Input: part model. Units: mm. Frame: model coordinates. Face numbers are marked on the shaded views. Give positions to 0.01 mm unless a question says otherwise; leave off trailing zeros. Loops run counter-clockwise (first coordinate to the right, second up) from the corner with the lowest first, then second, coordinate; pieces in that order, holes last. Notation, with made-up numbers: (54, 80.5) - (75, 80.5) arc R35 ccw to (75, 115.5) - close; hole circle Ø6 at (68.5, -36). An arc over 180 degrees is marked (long way). Answer as a JSON object with one key per item and string values. Group by question number.
(1) Section query C-C (z = -7). Return loops of the section in (x, y) (3 decimals), plus the area to 3 significant figures.
(2) Section query D-D (z = -17.5). Return loops of the section in (x, y), plus the area to 3 significant figures.
(3) Pin query (flat end, axial travel): P1, Ø3, axis at x = 0, z = 0, coming from the -Y side; P2, Ø1, axis at x = 3.5, y = 6.5, coming from the +Z side; P3, Ø3, axis at x = -15.5, z = 3.5, coming from the -Y side; P4, Ø4, axis at y = 4, z = 4, coming from the +X side. Return the tip coordinate at first contact, or that it passes through.
(4) Section query A-A (y = 3.5). Return loops of the section in (x, z).
(5) Material intervals for L1, parallel to X at y = 5.75, z = 0; L2, parallel to X at y = 2.75, z = 0; L3, parallel to Y at x = -14.5, z = -1, sorted ascending.
(6) Mould query, pull axis X, two halves, no side actions, for the marked faces 1 and 2. Classes: +X half, -X half, draft (parallel to the pull), parting line (faces both ways), or undercut.
(7) Section query B-B (x = 22). Return loops of the section in (y, z), plus the area to 3 significant figures.
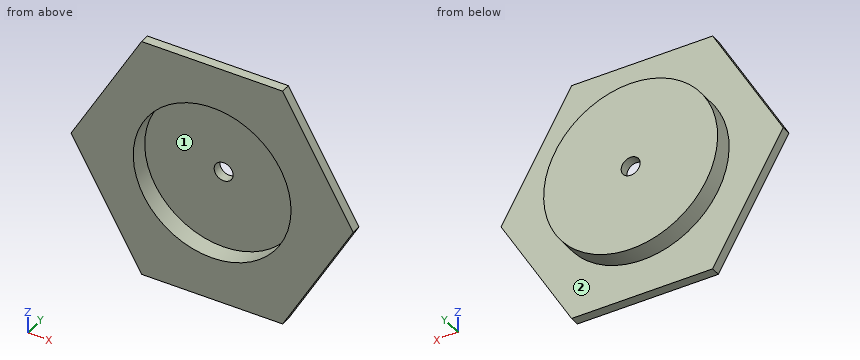
```python
from build123d import *

# Parameters (mm, degrees)
BOSS_EXTRUDE1_DEPTH = 2.5
SKETCH3_R           = 2.5
CUT_EXTRUDE1_DEPTH  = 2.5
SKETCH4_R           = 22.966828386
BOSS_EXTRUDE2_DEPTH = 5
SKETCH5_R           = 20.826616742
CUT_EXTRUDE2_DEPTH  = 5
SKETCH6_R           = 2.5
CUT_EXTRUDE3_DEPTH  = 5


with BuildPart() as part:
    # Sketch2 → Boss-Extrude1 (new body)
    with BuildSketch(Plane(origin=(0, 0, 0), x_dir=(1, 0, 0), z_dir=(0, 1, 0))):
        Polygon((37.25, 0), (18.625, 32.259446291), (-18.625, 32.259446291), (-37.25, 0), (-18.625, -32.259446291), (18.625, -32.259446291), align=None)
    extrude(amount=BOSS_EXTRUDE1_DEPTH)

    # Sketch3 → Cut-Extrude1 (cut)
    with BuildSketch(Plane.XZ):
        with Locations(Location((0, 0, 0), (0, 0, 270))):
            Circle(SKETCH3_R)
    extrude(amount=-CUT_EXTRUDE1_DEPTH, mode=Mode.SUBTRACT)

    # Sketch4 → Boss-Extrude2 (add)
    with BuildSketch(Plane(origin=(0, 2.5, 0), x_dir=(1, 0, 0), z_dir=(0, 1, 0))):
        with Locations(Location((0, 0, 0), (0, 0, 270))):
            Circle(SKETCH4_R)
    extrude(amount=BOSS_EXTRUDE2_DEPTH)

    # Sketch5 → Cut-Extrude2 (cut)
    with BuildSketch(Plane.XZ):
        with Locations(Location((0, 0, 0), (0, 0, 270))):
            Circle(SKETCH5_R)
    extrude(amount=-CUT_EXTRUDE2_DEPTH, mode=Mode.SUBTRACT)

    # Sketch6 → Cut-Extrude3 (cut)
    with BuildSketch(Plane.XZ.offset(-5)):
        with Locations(Location((0, 0, 0), (0, 0, 270))):
            Circle(SKETCH6_R)
    extrude(amount=-CUT_EXTRUDE3_DEPTH, mode=Mode.SUBTRACT)


solid = part.part
```
Recorded:
{
 "1": {"outline": "(-33.209, 0) - (-19.615, 0) - (-19.615, 5) - (19.615, 5) - (19.615, 0) - (33.209, 0) - (33.209, 2.5) - (21.874, 2.5) - (21.874, 7.5) - (-21.874, 7.5) - (-21.874, 2.5) - (-33.209, 2.5) - close", "area": "189 mm^2"},
 "2": {"outline": "(-27.15, 0) - (-11.29, 0) - (-11.29, 5) - (11.29, 5) - (11.29, 0) - (27.15, 0) - (27.15, 2.5) - (14.87, 2.5) - (14.87, 7.5) - (-14.87, 7.5) - (-14.87, 2.5) - (-27.15, 2.5) - close", "area": "172 mm^2"},
 "3": {"P1": "passes through", "P2": "stops at z = 22.77", "P3": "stops at y = 5", "P4": "stops at x = 35.7"},
 "4": {"outline": "circle Ø45.93 at (0, 0); hole circle Ø41.65 at (0, 0)"},
 "5": {"L1": "x = -22.97 to -2.5, 2.5 to 22.97", "L2": "x = -22.97 to -20.83, 20.83 to 22.97", "L3": "y = 5 to 7.5"},
 "6": {"face 1": "undercut", "face 2": "draft"},
 "7": {"outline": "(0, -26.41) - (2.5, -26.41) - (2.5, -6.59) - (7.5, -6.59) - (7.5, 6.59) - (2.5, 6.59) - (2.5, 26.41) - (0, 26.41) - close", "area": "198 mm^2"}
}
